Input: part model. Units: mm. Frame: model coordinates. A direction names the side the tool comes from. Coordinates: 2 decimals unless noted, no trailing zeros. Write each loop counter-clockwise with the first axis right and the second up, starting at its lowest first coordinate (ties: lowest second). Pieces come first, ordered by that corner, then holes. Notation, with made-up numbers: (85, 47) -> (112, 47) arc R34 cw to (112, 83) -> close; hole circle Ø6 at (52, 40). An arc over 180 degrees is marked (long way). Use one line per item in the form item = value. Start each with the question number.
(1) Set-up query: faces 5 (the face through (-9.704, -7.605, -16.128)), 6 (the face through (-50, 385, 117)), 7 (the face through (65, 222, 1)), 8 (the face through (95, 385, 1)), 9 (the face through (55, 385, 93)). Return all of +Z, -Z, +X, -X, +Y, -Y with unobstructed straight access to the full face (end or side cutting, diameter ignored); none if empty.
(2) First-contact query: pin 1 (6 mm diameter, centred on y = 390, z = 88.5, fed in from +X); pin 2 (11 mm diameter, centred on x = 80, y = 389.5, fed in from +Z); pin 3 (12 mm diameter, centred on y = 267, z = -50.5, fed in from +X). Flat tips, straight axial feed; report the tip coordinate or a pass-through.
(3) Cut plane B-B on x = 59.5. Return the cut outline in (y, z), plus the area to 3 significant figures.
(4) Pull-direction query (Y, two-part tool) for faces 1 (the face through (8.98, 396.67, 7.46)), 2 (the face through (-75, 228, 1)), 3 (the face through (-1, -15, -1)), 4 (the face through (25, 12, -43)); classes: released by +Y, released by -Y, zero draft, split by the parting line, or undercut.
(5) Cut plane A-A on y = 420. Return the cut outline in (x, z), plus the area to 3 significant figures.
(6) Ray query, line 1 along X through (y, z) = (20.5, -47); line 2 along Z through (x, y) = (-35, -3.5); line 3 along Z through (x, y) = (60.5, 432.5). Return the intervals inside material, ascending.
(7) Cut plane D-D on y = 359. Return the cut outline in (x, z), plus the area to 3 significant figures.
(8) Cut plane C-C on z = -38. Return the cut outline in (x, y), plus the area to 3 significant figures.
```python
from build123d import *

# Parameters (mm, degrees)
SKETCH2_W            = 150
SKETCH2_H            = 150
SKETCH2_W_2          = 130
SKETCH2_H_2          = 130
BOSS_EXTRUDE2_DEPTH  = 450
SKETCH4_W            = 150
SKETCH4_H            = 150
BOSS_EXTRUDE3_DEPTH  = 15
BOSS_EXTRUDE4_START  = -450
SKETCH4_2_W          = 150
SKETCH4_2_H          = 150
BOSS_EXTRUDE4_DEPTH  = 15
SKETCH5_R            = 30
CUT_EXTRUDE1_DEPTH   = 15
SKETCH7_W            = 20
SKETCH7_H            = 10
BOSS_EXTRUDE5_DEPTH  = 50
BOSS_EXTRUDE6_START  = -10
SKETCH9_R            = 25
BOSS_EXTRUDE6_DEPTH  = 20
CUT_EXTRUDE3_START   = 5
SKETCH10_R           = 25
SKETCH10_R_2         = 22
CUT_EXTRUDE3_DEPTH   = 10
SKETCH12_W           = 20
SKETCH12_H           = 40
BOSS_EXTRUDE7_DEPTH  = 25
SKETCH13_R           = 4
BOSS_EXTRUDE8_DEPTH  = 23
SKETCH18_W           = 110
SKETCH18_H           = 20
BOSS_EXTRUDE11_DEPTH = 20
CHAMFER1_SIZE        = 10
CHAMFER2_SIZE        = 10
SKETCH19_W           = 110
SKETCH19_H           = 20
BOSS_EXTRUDE12_DEPTH = 47
CHAMFER3_SIZE        = 10


with BuildPart() as part:
    # Sketch2 → Boss-Extrude2 (new body)
    with BuildSketch(Plane(origin=(0, 0, 0), x_dir=(1, 0, 0), z_dir=(0, 1, 0))):
        Rectangle(SKETCH2_W, SKETCH2_H)
        Rectangle(SKETCH2_W_2, SKETCH2_H_2, mode=Mode.SUBTRACT)
    extrude(amount=BOSS_EXTRUDE2_DEPTH)

    # Sketch4 → Boss-Extrude3 (add)
    with BuildSketch(Plane(origin=(0, 450, 0), x_dir=(1, 0, 0), z_dir=(0, 1, 0))):
        Rectangle(SKETCH4_W, SKETCH4_H)
    extrude(amount=BOSS_EXTRUDE3_DEPTH)

    # Sketch4_2 → Boss-Extrude4 (add)
    with BuildSketch(Plane(origin=(0, 450, 0), x_dir=(1, 0, 0), z_dir=(0, 1, 0)).offset(BOSS_EXTRUDE4_START)):
        Rectangle(SKETCH4_2_W, SKETCH4_2_H)
    extrude(amount=-BOSS_EXTRUDE4_DEPTH)

    # Sketch5 → Cut-Extrude1 (cut)
    with BuildSketch(Plane.XZ.offset(15)):
        with Locations(Location((-35, 0, 0), (0, 0, 270))):
            Circle(SKETCH5_R)
    extrude(amount=-CUT_EXTRUDE1_DEPTH, mode=Mode.SUBTRACT)

    # Sketch7 → Boss-Extrude5 (add)
    with BuildSketch(Plane.XZ.offset(-450)):
        with Locations((0, -15)):
            Rectangle(SKETCH7_W, SKETCH7_H)
    boss_extrude5 = extrude(amount=BOSS_EXTRUDE5_DEPTH)

    # Mirror1: Boss-Extrude5 across plane
    add(boss_extrude5.mirror(Plane.XY))

    # Sketch9 → Boss-Extrude6 (add)
    with BuildSketch(Plane.XY.offset(BOSS_EXTRUDE6_START)):
        with Locations(Location((0, 420, 0), (0, 0, 113.578178478))):
            Circle(SKETCH9_R)
    extrude(amount=BOSS_EXTRUDE6_DEPTH)

    # Sketch10 → Cut-Extrude3 (cut)
    with BuildSketch(Plane.XY.offset(-10).offset(CUT_EXTRUDE3_START)):
        with Locations(Location((0, 420, 0), (0, 0, 113.578178478))):
            Circle(SKETCH10_R)
        with Locations((0, 420)):
            Circle(SKETCH10_R_2, mode=Mode.SUBTRACT)
    extrude(amount=CUT_EXTRUDE3_DEPTH, mode=Mode.SUBTRACT)

    # Sketch12 → Boss-Extrude7 (add)
    with BuildSketch(Plane(origin=(0, 0, 0), x_dir=(1, 0, 0), z_dir=(0, 1, 0))):
        with Locations((35, 43)):
            Rectangle(SKETCH12_W, SKETCH12_H)
    extrude(amount=BOSS_EXTRUDE7_DEPTH)

    # Sketch13 → Boss-Extrude8 (add)
    with BuildSketch(Plane.XY.offset(-23)):
        with Locations(Location((35.121485498, 12.610702381, 0), (0, 0, 180))):
            Circle(SKETCH13_R)
    extrude(amount=BOSS_EXTRUDE8_DEPTH)

    # Sketch18 → Boss-Extrude11 (add)
    with BuildSketch(Plane(origin=(75, 0, 0), x_dir=(0, 0, -1), z_dir=(1, 0, 0))):
        with Locations((0, 385)):
            Rectangle(SKETCH18_W, SKETCH18_H)
    extrude(amount=BOSS_EXTRUDE11_DEPTH)

    # Chamfer1
    chamfer1_edges = [part.edges().sort_by_distance(p)[0] for p in [
        (95, 385, 55),
    ]]
    chamfer(chamfer1_edges, length=CHAMFER1_SIZE)

    # Chamfer2
    chamfer2_edges = [part.edges().sort_by_distance(p)[0] for p in [
        (95, 385, -55),
    ]]
    chamfer(chamfer2_edges, length=CHAMFER2_SIZE)

    # Sketch19 → Boss-Extrude12 (add)
    with BuildSketch(Plane.XY.offset(75)):
        with Locations((0, 385)):
            Rectangle(SKETCH19_W, SKETCH19_H)
    extrude(amount=BOSS_EXTRUDE12_DEPTH)

    # Chamfer3
    chamfer3_edges = [part.edges().sort_by_distance(p)[0] for p in [
        (-55, 385, 122),
        (55, 385, 122),
    ]]
    chamfer(chamfer3_edges, length=CHAMFER3_SIZE)


solid = part.part
```
Values:
q1.face_5 = -Y
q1.face_6 = +Z, -X, +Y, -Y
q1.face_7 = none
q1.face_8 = +Z, -Z, +X, +Y, -Y
q1.face_9 = +Z, +X, +Y, -Y
q2.pin_1 = 55
q2.pin_2 = 75
q2.pin_3 = 75
q3.outline = (-15, -75) -> (465, -75) -> (465, 75) -> (-15, 75) -> close; hole (0, -65) -> (450, -65) -> (450, 65) -> (0, 65) -> close
q3.area = 13,500 mm2
q4.face_1 = undercut
q4.face_2 = zero draft
q4.face_3 = released by -Y
q4.face_4 = undercut
q5.outline = (-75, -75) -> (75, -75) -> (75, 75) -> (-75, 75) -> close; (-25, -10) -> (-10, -10) -> (-10, -20) -> (10, -20) -> (10, -10) -> (25, -10) -> (25, -5) -> (22, -5) -> (22, 5) -> (25, 5) -> (25, 10) -> (10, 10) -> (10, 20) -> (-10, 20) -> (-10, 10) -> (-25, 10) -> (-25, 5) -> (-22, 5) -> (-22, -5) -> (-25, -5) -> close; hole (-65, -65) -> (65, -65) -> (65, 65) -> (-65, 65) -> close
q5.area = 6,940 mm2
q6.line_1 = -75 to -65, 25 to 45, 65 to 75
q6.line_2 = -75 to -30, 30 to 75
q6.line_3 = -75 to -65, 65 to 75
q7.outline = (-75, -75) -> (75, -75) -> (75, 75) -> (-75, 75) -> close; hole (-65, -65) -> (65, -65) -> (65, 65) -> (-65, 65) -> close
q7.area = 5,600 mm2
q8.outline = (-75, -15) -> (75, -15) -> (75, 375) -> (95, 375) -> (95, 395) -> (75, 395) -> (75, 465) -> (-75, 465) -> close; hole (-65, 0) -> (25, 0) -> (25, 25) -> (45, 25) -> (45, 0) -> (65, 0) -> (65, 450) -> (-65, 450) -> close
q8.area = 14,400 mm2
